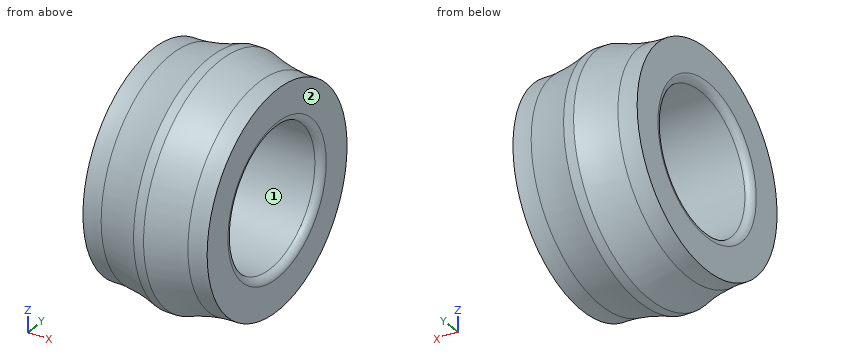
Autodesk Inventor part; units mm, degrees
ref_plane "NO_GEO_XY" through (0, 0, 0) normal (1, 0, 0) x (0, 0, -1)
ref_plane "NO_GEO_YZ" through (0, 0, 0) normal (0, 0, -1) x (0, 1, 0)
ref_plane "NO_GEO_ZX" through (0, 0, 0) normal (0, 1, 0) x (1, 0, 0)
sketch "Sketch_1" plane through (0, 0, 0) normal (0, 0, 1) x (1, 0, 0)
  line L0 (18, 0) -> (-18, 0)
  arc A0 (0, 11) -> (1, 10) centre (1, 11) ccw
  line L1 (1, 10) -> (17, 10)
  arc A1 (17, 10) -> (18, 11) centre (17, 11) ccw
  line L2 (18, 11) -> (18, 15.65)
  arc A2 (15.289, 15.7632) -> (18, 15.65) centre (17.3933, 33.6398) ccw
  arc A3 (9.7224, 17.0927) -> (15.289, 15.7632) centre (17.8763, 38.9136) ccw
  line L3 (9.7224, 17.0927) -> (8.2776, 17.0927)
  arc A4 (2.711, 15.7632) -> (8.2776, 17.0927) centre (0.1237, 38.9136) ccw
  arc A5 (0, 15.65) -> (2.711, 15.7632) centre (0.6067, 33.6398) ccw
  line L4 (0, 15.65) -> (0, 11)
revolve "Revolution1" add sketch "Sketch_1" angle 360 about axis through (18, 0, 0) along (1, 0, 0)
ref_plane "NO_GEO_XY" through (0, 0, 0) normal (1, 0, 0) x (0, 0, -1)
ref_plane "NO_GEO_YZ" through (0, 0, 0) normal (0, 0, -1) x (0, 1, 0)
ref_plane "NO_GEO_ZX" through (0, 0, 0) normal (0, 1, 0) x (1, 0, 0)
ref_plane "ir_XY" through (0, 0, 0) normal (0, 0, 1) x (1, 0, 0)
ref_plane "ir_YZ" through (0, 0, 0) normal (1, 0, 0) x (0, 1, 0)
ref_plane "ir_ZX" through (0, 0, 0) normal (0, 1, 0) x (0, 0, 1)
properties part number "22205/20 E_ir"
Can you work these out from the model? Positions are in its coordinate system, mm. Face numbers are marked on the shaded views. Coordinates: 2 decimals unless noted, no trailing zeros. Loops run counter-clockwise (first coordinate to the right, second up) from the corner with the lowest first, then second, coordinate; pieces in that order, holes last. Notation, with made-up numbers: (57.25, 24) - (111.25, 24) arc R15 cw to (111.25, 42) - close; hole circle Ø7 at (-11, 23.5). An arc over 180 degrees is marked (long way). Put each result on its own line as item: value. Start each with the question number.
Item 1: If I drill on line 1 along Y through (x, z) = (8.75, 1); line 2 along Y through (x, z) = (2.25, -6.5); line 3 along Z through (x, y) = (9.75, 0), over which ranges is the centre line in solid material (lowest first)?
Item 2: Suppose I cut it at D-D (x = 6.75). Please give me the cut outline in (y, z), and give its area (3 significant figures).
Item 3: Suppose I cut it at C-C (x = 8.75). Please give me the cut outline in (y, z).
Item 4: Suppose I cut it at A-A (y = 0). Please give me the cut outline in (x, z), and give its area (3 significant figures).
Item 5: For pin 1 (10 mm diameter, centred on x = 12.5, y = -6.5, fed in from +Z); pin 2 (2 mm diameter, centred on x = 4, z = 12, fed in from +Y); pin 3 (8 mm diameter, centred on y = -3.5, z = -7.5, fed in from +X); pin 4 (5 mm diameter, centred on x = 14.5, y = 7, fed in from +Z), each with a flat end and sliding along its axis, tell me the tip position at first contact or that it passes through.
Item 6: If we mould it in two halves opening along Y, with no side actions, what happens to the marked faces 1 and 2? For each: +Y half, -Y half, draft (parallel to the pull), parting line (faces both ways), or undercut.
Here are the results:
1. line 1: -17.06 to -9.95, 9.95 to 17.06
1. line 2: -14.31 to -7.6, 7.6 to 14.31
1. line 3: -17.08 to -10, 10 to 17.08
2. outline: circle Ø33.16 at (0, 0); hole circle Ø20 at (0, 0)
2. area: 550 mm²
3. outline: circle Ø34.19 at (0, 0); hole circle Ø20 at (0, 0)
4. outline: (0, -15.65) arc R18 cw to (2.71, -15.76) arc R23.3 cw to (8.28, -17.09) - (9.72, -17.09) arc R23.29 cw to (15.29, -15.76) arc R18 cw to (18, -15.65) - (18, -11) arc R1 ccw to (17, -10) - (1, -10) arc R1 ccw to (0, -11) - close; (0, 11) arc R1 ccw to (1, 10) - (17, 10) arc R1 ccw to (18, 11) - (18, 15.65) arc R18 cw to (15.29, 15.76) arc R23.29 cw to (9.72, 17.09) - (8.28, 17.09) arc R23.3 cw to (2.71, 15.76) arc R18 cw to (0, 15.65) - close
4. area: 222 mm²
5. pin 1: z = 16.93
5. pin 2: y = 11.57
5. pin 3: x = 18
5. pin 4: z = 15.34
6. face 1: undercut
6. face 2: draft
